Geometry check sheet. Reference: the model listing, model coordinates, mm. Coordinates: 2 decimals unless noted, no trailing zeros. Write each loop counter-clockwise with the first axis right and the second up, starting at its lowest first coordinate (ties: lowest second). Pieces come first, ordered by that corner, then holes.
from build123d import *

# Parameters (mm, degrees)
F1_DEPTH = 19.05
F2_R     = 25.4
F3_R     = 4.7879
F4_DEPTH = 33.02
F5_R     = 3.96875
F6_DEPTH = 28.575


# Not quite as in the source:
# - a feature names something its author has since deleted; it is built from what else it names


with BuildPart() as f1:
    # F0 (on Front) → F1 (new body)
    with BuildSketch(Plane.XZ):
        with BuildLine():
            Line((-266.7, -63.5), (-266.7, -88.9))
            Line((-266.7, -88.9), (266.7, -88.9))
            Line((266.7, -88.9), (266.7, -63.5))
            Line((266.7, -63.5), (245.919625, -63.5))
            ThreePointArc((245.919625, -63.5), (241.249891817, -61.565733183), (239.315625, -56.896))
            Line((239.315625, -56.896), (239.315625, 0))
            Line((239.315625, 0), (266.7, 50.8))
            Line((266.7, 50.8), (266.7, 88.9))
            Line((266.7, 88.9), (-266.7, 88.9))
            Line((-266.7, 88.9), (-266.7, 50.8))
            Line((-266.7, 50.8), (-239.315625, 0))
            Line((-239.315625, 0), (-239.315625, -56.896))
            ThreePointArc((-239.315625, -56.896), (-241.249891817, -61.565733183), (-245.919625, -63.5))
            Line((-245.919625, -63.5), (-266.7, -63.5))
        make_face()
        with BuildLine():
            Line((-63.5, -63.5), (-88.9, -63.5))
            ThreePointArc((-88.9, -63.5), (-97.8802561211, -59.7802561211), (-101.6, -50.8))
            Line((-101.6, -50.8), (-101.6, -9.525))
            ThreePointArc((-101.6, -9.525), (-95.0904482119, 6.1904482119), (-79.375, 12.7))
            Line((-79.375, 12.7), (-73.025, 12.7))
            ThreePointArc((-73.025, 12.7), (-57.3095517881, 6.1904482119), (-50.8, -9.525))
            Line((-50.8, -9.525), (-50.8, -50.8))
            ThreePointArc((-50.8, -50.8), (-54.5197438789, -59.7802561211), (-63.5, -63.5))
        make_face(mode=Mode.SUBTRACT)
        with BuildLine():
            ThreePointArc((63.5, -63.5), (54.5197438789, -59.7802561211), (50.8, -50.8))
            Line((50.8, -50.8), (50.8, -9.525))
            ThreePointArc((50.8, -9.525), (57.3095517881, 6.1904482119), (73.025, 12.7))
            Line((73.025, 12.7), (79.375, 12.7))
            ThreePointArc((79.375, 12.7), (95.0904482119, 6.1904482119), (101.6, -9.525))
            Line((101.6, -9.525), (101.6, -50.8))
            ThreePointArc((101.6, -50.8), (97.8802561211, -59.7802561211), (88.9, -63.5))
            Line((88.9, -63.5), (63.5, -63.5))
        make_face(mode=Mode.SUBTRACT)
    extrude(amount=F1_DEPTH)

    # F2
    f2_edges = [f1.edges().sort_by_distance(p)[0] for p in [
        (-266.7, -9.525, 50.8),
        (-239.315625, -9.525, 0),
        (266.7, -9.525, 50.8),
        (239.315625, -9.525, 0),
    ]]
    fillet(f2_edges, radius=F2_R)

    # F3 (on face) → F4 (cut)
    with BuildSketch(Plane(origin=(0, 0, -88.9), x_dir=(1, 0, 0), z_dir=(0, 0, -1))):
        with Locations((-254, 9.525)):
            Circle(F3_R)
        with Locations((-76.2, 9.525)):
            Circle(F3_R)
        with Locations((254, 9.525)):
            Circle(F3_R)
        with Locations((76.2, 9.525)):
            Circle(F3_R)
    extrude(amount=-F4_DEPTH, mode=Mode.SUBTRACT)

    # F5 (on face) → F6 (cut)
    with BuildSketch(Plane.XY.offset(88.9)):
        with Locations((-254, -9.525)):
            Circle(F5_R)
        with Locations((-76.2, -9.525)):
            Circle(F5_R)
        with Locations((76.2, -9.525)):
            Circle(F5_R)
        with Locations((254, -9.525)):
            Circle(F5_R)
    extrude(amount=-F6_DEPTH, mode=Mode.SUBTRACT)


solid = f1.part
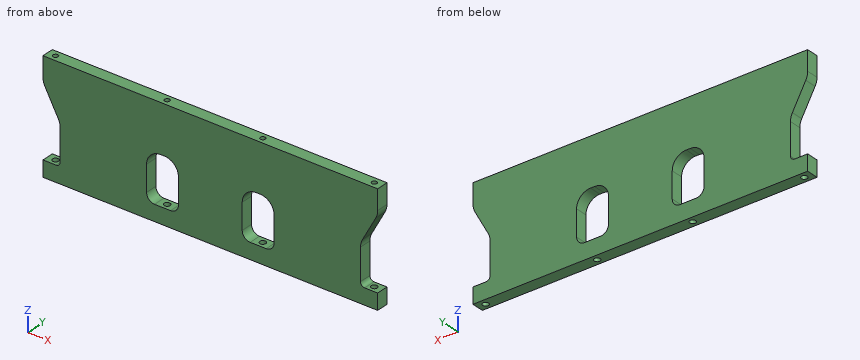
1. Gauge pin test, flat ends, axial feed: pin 1 Ø2 at (y, z) = (-10.5, -24.5) entering from +X; pin 2 Ø5 at (x, y) = (-76.2, -9.525) entering from -Z; pin 3 Ø9.5 at (y, z) = (-6.5, -29) entering from -X. Record the tip position at first contact, or that the pin passes through.
Computed values:
pin 1: stops at x = 239.32
pin 2: stops at z = 12.7
pin 3: stops at x = -239.32
2. Thickness scan on line 1 along X through (y, z) = (-9.25, -72.5); line 2 along X through (y, z) = (-17.5, -42); line 3 along Y through (x, z) = (-254, 69.25). Record the ranges inside material, lowest first.
Computed values:
line 1: x = -266.7 to -258.78, -249.22 to -80.98, -71.42 to 71.42, 80.98 to 249.22, 258.78 to 266.7
line 2: x = -239.32 to -101.6, -50.8 to 50.8, 101.6 to 239.32
line 3: y = -19.05 to -13.49, -5.56 to 0
3. Sectioned sample at A-A, the plane z = -75.5. Record the boundary of the cut face in (x, y) (3 decimals), and give its area (3 significant figures).
Computed values:
outline: (-266.7, -19.05) - (266.7, -19.05) - (266.7, 0) - (-266.7, 0) - close; hole circle Ø9.576 at (-254, -9.525); hole circle Ø9.576 at (-76.2, -9.525); hole circle Ø9.576 at (76.2, -9.525); hole circle Ø9.576 at (254, -9.525)
area: 9,870 mm2
4. Sectioned sample at B-B, the plane z = -30. Record the boundary of the cut face in (x, y).
Computed values:
outline: (-239.32, -19.05) - (-101.6, -19.05) - (-101.6, 0) - (-239.32, 0) - close; (-50.8, -19.05) - (50.8, -19.05) - (50.8, 0) - (-50.8, 0) - close; (101.6, -19.05) - (239.32, -19.05) - (239.32, 0) - (101.6, 0) - close
5. Sectioned sample at C-C, the plane z = 36. Record the boundary of the cut face in (x, y).
Computed values:
outline: (-258.72, -19.05) - (258.72, -19.05) - (258.72, 0) - (-258.72, 0) - close
